from build123d import *

# Parameters (mm, degrees)
CYLINDER010_R     = 2
CYLINDER010_DEPTH = 3
CYLINDER_R        = 38
CYLINDER_DEPTH    = 20
CYLINDER001_R     = 40
CYLINDER001_DEPTH = 19


with BuildPart() as wirehole:
    # Cylinder010 → Cylinder010 (new body)
    with BuildSketch(Plane(origin=(38, 1, 5), x_dir=(1, 0, 0), z_dir=(0, -1, 0))):
        Circle(CYLINDER010_R)
    extrude(amount=CYLINDER010_DEPTH)


with BuildPart() as obj1:
    # Cylinder → Cylinder (new body)
    with BuildSketch(Plane(origin=(38, 38, -1), x_dir=(1, 0, 0), z_dir=(0, 0, 1))):
        Circle(CYLINDER_R)
    extrude(amount=CYLINDER_DEPTH)

    # Fusion004: union WireHole
    add(wirehole.part)


with BuildPart() as depth:
    # Cylinder001 → Cylinder001 (new body)
    with BuildSketch(Plane(origin=(38, 38, -1), x_dir=(1, 0, 0), z_dir=(0, 0, 1))):
        Circle(CYLINDER001_R)
    extrude(amount=CYLINDER001_DEPTH)

    # Cut007: cut obj1
    add(obj1.part, mode=Mode.SUBTRACT)


with BuildPart() as depth_1:
    # Cut007 placement: moved
    add(depth.part.moved(Location((0, 2, 2))))


solid = depth_1.part
Geometry: final body of the model. Coordinates: model frame, mm. Give positions to 0.01 mm unless a question says otherwise; leave off trailing zeros. Write each loop counter-clockwise with the first axis right and the second up, starting at its lowest first coordinate (ties: lowest second). Pieces come first, ordered by that corner, then holes. Notation, with made-up numbers: (-30.75, -11) - (10.25, -11) arc R22 cw to (10.25, 20) - close; hole circle Ø9 at (-14, 87). An arc over 180 degrees is marked (long way). Return JSON: item names as keys, results as strings. Group by question number.
1) Section D-D on z = 12. Return the cut outline in (x, y).
2) Section B-B on y = 40. Return the cut outline in (x, z), plus the area to 3 significant figures.
3) Mould query, pull axis Z, two halves, no side actions, for faces 1 (the flat face through (52.6, 4.6, 20)), 2 (the cylindrical face through (36, 1, 7)), 3 (the flat face through (52.6, 4.6, 1)). Classes: released by +Z, released by -Z, zero draft, split by the parting line, or undercut.
4) First-contact query: P1, Ø2.5, axis at x = 38, z = 7, coming from the -Y side; P2, Ø4, axis at x = 39, z = 5, coming from the +Y side; P3, Ø5, axis at x = 49.5, z = 7.5, coming from the +Y side. Flat tips, straight axial feed; report the tip coordinate or a pass-through.
5) Section A-A on x = 38. Return the cut outline in (y, z).
6) Section C-C on x = 56. Return the cut outline in (y, z).
7) Line query: line 1 (Z direction, x = 38, y = 1); line 2 (Y direction, x = 38, z = 16); line 3 (Y direction, x = 38, z = 8.5). Output: solid intervals per line, ascending.
Filled in:
{
 "1": {"outline": "circle Ø80 at (38, 40); hole circle Ø76 at (38, 40)"},
 "2": {"outline": "(-2, 1) - (0, 1) - (0, 20) - (-2, 20) - close; (76, 1) - (78, 1) - (78, 20) - (76, 20) - close", "area": "76.0 mm^2"},
 "3": {"face 1": "released by +Z", "face 2": "undercut", "face 3": "released by -Z"},
 "4": {"P1": "stops at y = 77.98", "P2": "stops at y = 80", "P3": "stops at y = 78.97"},
 "5": {"outline": "(0, 1) - (2, 1) - (2, 5) - (0, 5) - close; (0, 9) - (2, 9) - (2, 20) - (0, 20) - close; (78, 1) - (80, 1) - (80, 20) - (78, 20) - close"},
 "6": {"outline": "(4.28, 1) - (6.53, 1) - (6.53, 20) - (4.28, 20) - close; (73.47, 1) - (75.72, 1) - (75.72, 20) - (73.47, 20) - close"},
 "7": {"line 1": "z = 1 to 5, 9 to 20", "line 2": "y = 0 to 2, 78 to 80", "line 3": "y = 78 to 80"}
}
